Part model, mm, in its own coordinate system. Face numbers are marked on the shaded views. A direction names the side the tool comes from. Round coordinates to 2 decimals unless told otherwise and drop trailing zeros. Write each loop counter-clockwise with the first axis right and the second up, starting at its lowest first coordinate (ties: lowest second). Pieces come first, ordered by that corner, then holes. Notation, with made-up numbers: M 26.5,2.5 L 80.5,2.5 A15 cw 80.5,14.5 Z; hole C -9.5,-35.75 d7. An arc over 180 degrees is marked long. Answer as a JSON object with one key per item and string values. Group by question number.
1. Band-saw the part on D-D, the plane x = -11. Write the cut outline in (y, z), plus the area to 3 significant figures.
2. Band-saw the part on A-A, the plane y = -56.5. Write the cut outline in (x, z).
3. Drop flat-ended pins along their axis: pin 1 (5 mm diameter, centred on x = -11, z = 34, fed in from -Y); pin 2 (4 mm diameter, centred on x = -23.5, y = -55.5, fed in from +Z); pin 3 (6 mm diameter, centred on x = -8.5, y = -39.5, fed in from +Z); pin 4 (2.5 mm diameter, centred on y = -56.5, z = 30, fed in from -X). Give the stop position or say it passes through.
4. Which spindle directions (+Z, -Z, +X, -X, +Y, -Y) get a long thin tool onto all of the face, cutting with end or side? Do the marked faces 1, 2, 3 and 4. Say none if no direction does.
5. Band-saw the part on C-C, the plane x = 26. Write the cut outline in (y, z).
6. Two-plate mould, pull along Y, no slides. Class the marked faces 5, 6, 7 and 8: +Y half, -Y half, draft (parallel to the pull), parting line (faces both ways), or undercut.
7. Drill centre lines: line 1 (Z direction, x = 42.35, y = -13); line 2 (Z direction, x = -11, y = -37.5); line 3 (X direction, y = -1.6, z = 65). Where is each one in solid material? Low to high. Write a range as from..to.
8. Band-saw the part on B-B, the plane z = 17. Write the cut outline in (x, y).
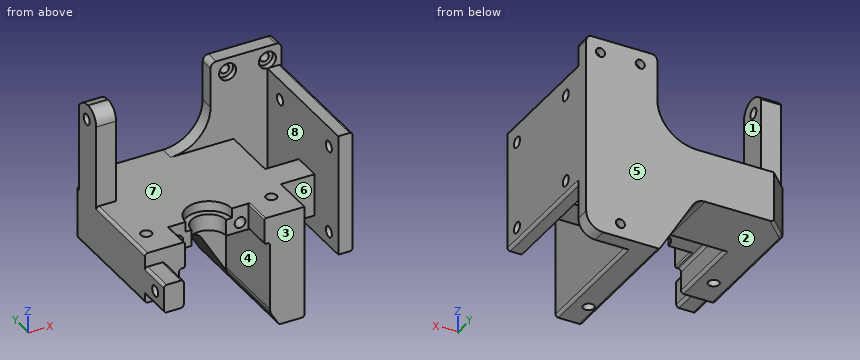
from build123d import *

# Parameters (mm, degrees)
PAD_DEPTH       = 70
SKETCH001_W     = 11.887794
SKETCH001_H     = 46.78
POCKET_DEPTH    = 70.001
POCKET001_DEPTH = 30
SKETCH003_R     = 1.9
POCKET002_DEPTH = 40.001
POCKET003_DEPTH = 3.5
POCKET004_DEPTH = 9
SKETCH021_W     = 28
SKETCH021_H     = 53.161749
POCKET005_DEPTH = 10
SKETCH022_W     = 32
SKETCH022_H     = 58.660217
POCKET006_DEPTH = 28
POCKET007_DEPTH = 51
SKETCH008_W     = 19.05323
SKETCH008_H     = 10.69447
SKETCH008_W_2   = 35.750058
SKETCH008_H_2   = 36.172176
POCKET008_DEPTH = 45
SKETCH009_R     = 1.9
POCKET009_DEPTH = 5
SKETCH015_W     = 11
SKETCH015_H     = 38.184422
SKETCH015_W_2   = 19.881198
SKETCH015_H_2   = 10
PAD001_DEPTH    = 7
SKETCH011_R     = 1.9
POCKET010_DEPTH = 10
SKETCH014_W     = 10
SKETCH014_H     = 15
PAD002_DEPTH    = 18
SKETCH010_R     = 1.6
POCKET011_DEPTH = 6
SKETCH017_R     = 3
POCKET012_DEPTH = 2
SKETCH013_R     = 1.9
POCKET013_DEPTH = 10
CHAMFER_SIZE    = 7
CHAMFER001_SIZE = 3
FILLET_R        = 6
FILLET001_R     = 5
FILLET002_R     = 1
FILLET003_R     = 1
FILLET004_R     = 1
FILLET005_R     = 1
FILLET006_R     = 5
FILLET007_R     = 4
FILLET008_R     = 1
FILLET009_R     = 1
FILLET010_R     = 1
FILLET011_R     = 0.5
FILLET012_R     = 1
FILLET013_R     = 1
FILLET014_R     = 1
FILLET015_R     = 14
FILLET016_R     = 2
FILLET017_R     = 6
FILLET018_R     = 1


with BuildPart() as part:
    # Sketch → Pad (new body)
    with BuildSketch(Plane.XY):
        Polygon((0, 0), (45, 0), (45, -50), (-28, -50), (-28, 0), align=None)
    extrude(amount=PAD_DEPTH)

    # Sketch001 (on Face7 of Pad) → Pocket (cut, through all)
    with BuildSketch(Plane.XY.offset(70)):
        with Locations((34.056103, -28.39)):
            Rectangle(SKETCH001_W, SKETCH001_H)
    extrude(amount=-POCKET_DEPTH, mode=Mode.SUBTRACT)

    # Sketch002 (on Face5 of Pocket) → Pocket001 (cut)
    with BuildSketch(Plane.XY.offset(70)):
        Polygon((30, -5), (30, -65.096024), (-40.783405, -65.096024), (-40.783405, 12.994774), (20, 12.994774), (20, -5), align=None)
    extrude(amount=-POCKET001_DEPTH, mode=Mode.SUBTRACT)

    # Sketch003 (on Face6 of Pocket001) → Pocket002 (cut, through all)
    with BuildSketch(Plane.XY.offset(40)):
        with Locations((-22, -40)):
            Circle(SKETCH003_R)
        with Locations((22, -40)):
            Circle(SKETCH003_R)
    extrude(amount=-POCKET002_DEPTH, mode=Mode.SUBTRACT)

    # Sketch004 (on Face6 of Pocket002) → Pocket003 (cut)
    with BuildSketch(Plane.XY.offset(40)):
        with BuildLine():
            ThreePointArc((8.125, -40), (0, -31.875), (-8.125, -40))
            Line((-8.125, -59.24), (-8.125, -40))
            Line((8.125, -59.24), (-8.125, -59.24))
            Line((8.125, -40), (8.125, -59.24))
        make_face()
    extrude(amount=-POCKET003_DEPTH, mode=Mode.SUBTRACT)

    # Sketch018 → Pocket004 (cut)
    with BuildSketch(Plane.XY.offset(36.5)):
        with BuildLine():
            ThreePointArc((6.1, -40), (0, -33.9), (-6.1, -40))
            Line((-6.1, -40), (-6.1, -58.98))
            Line((6.1, -58.98), (-6.1, -58.98))
            Line((6.1, -40), (6.1, -58.98))
        make_face()
    extrude(amount=-POCKET004_DEPTH, mode=Mode.SUBTRACT)

    # Sketch021 (on Face9 of Pocket004) → Pocket005 (cut)
    with BuildSketch(Plane.XZ.offset(50)):
        with Locations((0, 16.83664)):
            Rectangle(SKETCH021_W, SKETCH021_H)
    extrude(amount=-POCKET005_DEPTH, mode=Mode.SUBTRACT)

    # Sketch022 (on Face13 of Pocket005) → Pocket006 (cut)
    with BuildSketch(Plane.XZ.offset(50)):
        with Locations((0, 1.369891)):
            Rectangle(SKETCH022_W, SKETCH022_H)
    extrude(amount=-POCKET006_DEPTH, mode=Mode.SUBTRACT)

    # Sketch023 (on Face9 of Pocket006) → Pocket007 (cut)
    with BuildSketch(Plane.XZ.offset(50)):
        Polygon((-38.33, 22), (6, 22), (24, -8), (-38.33, -8), align=None)
    extrude(amount=-POCKET007_DEPTH, mode=Mode.SUBTRACT)

    # Sketch008 (on Face14 of Pocket007) → Pocket008 (cut)
    with BuildSketch(Plane.XZ.offset(50)):
        with Locations((44.142395, 67.347235)):
            Rectangle(SKETCH008_W, SKETCH008_H)
        with Locations((52.797694, 0.913912)):
            Rectangle(SKETCH008_W_2, SKETCH008_H_2)
    extrude(amount=-POCKET008_DEPTH, mode=Mode.SUBTRACT)

    # Sketch009 (on Face3 of Pocket008) → Pocket009 (cut)
    with BuildSketch(Plane.YZ.offset(45)):
        with Locations((-44, 55)):
            Circle(SKETCH009_R)
        with Locations((-13, 24)):
            Circle(SKETCH009_R)
        with Locations((-13, 55)):
            Circle(SKETCH009_R)
        with Locations((-44, 24)):
            Circle(SKETCH009_R)
    extrude(amount=-POCKET009_DEPTH, mode=Mode.SUBTRACT)

    # Sketch015 (on Face27 of Pocket009) → Pad001 (join)
    with BuildSketch(Plane(origin=(-28, 0, 0), x_dir=(0, -1, 0), z_dir=(-1, 0, 0))):
        with Locations((13.5, 54.907789)):
            Rectangle(SKETCH015_W, SKETCH015_H)
        with Locations((52.059401, 30)):
            Rectangle(SKETCH015_W_2, SKETCH015_H_2)
    extrude(amount=-PAD001_DEPTH)

    # Sketch011 (on Face27 of Pad001) → Pocket010 (cut)
    with BuildSketch(Plane(origin=(-28, 0, 0), x_dir=(0, -1, 0), z_dir=(-1, 0, 0))):
        with Locations((56.5, 30)):
            Circle(SKETCH011_R)
        with Locations((13, 68.5)):
            Circle(SKETCH011_R)
    extrude(amount=-POCKET010_DEPTH, mode=Mode.SUBTRACT)

    # Sketch014 (on Face3 of Pocket010) → Pad002 (join)
    with BuildSketch(Plane.YZ.offset(45)):
        with Locations((-30, 32.5)):
            Rectangle(SKETCH014_W, SKETCH014_H)
    extrude(amount=-PAD002_DEPTH)

    # Sketch010 → Pocket011 (cut)
    with BuildSketch(Plane(origin=(0, 0, 0), x_dir=(-1, 0, 0), z_dir=(0, 1, 0))):
        with Locations((-33, 5)):
            Circle(SKETCH010_R)
        with Locations((-40, 65)):
            Circle(SKETCH010_R)
        with Locations((-26, 65)):
            Circle(SKETCH010_R)
    extrude(amount=-POCKET011_DEPTH, mode=Mode.SUBTRACT)

    # Sketch017 (on Face34 of Pocket011) → Pocket012 (cut)
    with BuildSketch(Plane.XZ.offset(5)):
        with Locations((26, 65)):
            Circle(SKETCH017_R)
        with Locations((33, 5)):
            Circle(SKETCH017_R)
        with Locations((40, 65)):
            Circle(SKETCH017_R)
    extrude(amount=-POCKET012_DEPTH, mode=Mode.SUBTRACT)

    # Sketch013 (on Face43 of Pocket012) → Pocket013 (cut)
    with BuildSketch(Plane.XZ.offset(40)):
        with Locations((-11, 34)):
            Circle(SKETCH013_R)
        with Locations((11, 34)):
            Circle(SKETCH013_R)
    extrude(amount=-POCKET013_DEPTH, mode=Mode.SUBTRACT)

    # Chamfer
    chamfer_edges = [part.edges().sort_by_distance(p)[0] for p in [
        (-28, 0, 31),
    ]]
    chamfer(chamfer_edges, length=CHAMFER_SIZE)

    # Chamfer001
    chamfer001_edges = [part.edges().sort_by_distance(p)[0] for p in [
        (-24.5, -8, 74),
    ]]
    chamfer(chamfer001_edges, length=CHAMFER001_SIZE)

    # Fillet
    fillet_edges = [part.edges().sort_by_distance(p)[0] for p in [
        (-24.5, -11, 74),
    ]]
    fillet(fillet_edges, radius=FILLET_R)

    # Fillet001
    fillet001_edges = [part.edges().sort_by_distance(p)[0] for p in [
        (-24.5, -19, 74),
    ]]
    fillet(fillet001_edges, radius=FILLET001_R)

    # Fillet002
    fillet002_edges = [part.edges().sort_by_distance(p)[0] for p in [
        (-28, -34.5, 40),
    ]]
    fillet(fillet002_edges, radius=FILLET002_R)

    # Fillet003
    fillet003_edges = [part.edges().sort_by_distance(p)[0] for p in [
        (-28, -28.5, 22),
    ]]
    fillet(fillet003_edges, radius=FILLET003_R)

    # Fillet004
    fillet004_edges = [part.edges().sort_by_distance(p)[0] for p in [
        (-16, -36, 22),
    ]]
    fillet(fillet004_edges, radius=FILLET004_R)

    # Fillet005
    fillet005_edges = [part.edges().sort_by_distance(p)[0] for p in [
        (19.2, -25, 0),
    ]]
    fillet(fillet005_edges, radius=FILLET005_R)

    # Fillet006
    fillet006_edges = [part.edges().sort_by_distance(p)[0] for p in [
        (6, -11, 22),
    ]]
    fillet(fillet006_edges, radius=FILLET006_R)

    # Fillet007
    fillet007_edges = [part.edges().sort_by_distance(p)[0] for p in [
        (16, -36, 5.333333),
    ]]
    fillet(fillet007_edges, radius=FILLET007_R)

    # Fillet008
    fillet008_edges = [part.edges().sort_by_distance(p)[0] for p in [
        (16, -36, 30.7),
    ]]
    fillet(fillet008_edges, radius=FILLET008_R)

    # Fillet009
    fillet009_edges = [part.edges().sort_by_distance(p)[0] for p in [
        (-16, -36, 30.7),
    ]]
    fillet(fillet009_edges, radius=FILLET009_R)

    # Fillet010
    fillet010_edges = [part.edges().sort_by_distance(p)[0] for p in [
        (-28, -56, 25),
        (-21, -56, 25),
        (-21, -56, 35),
        (-28, -56, 35),
    ]]
    fillet(fillet010_edges, radius=FILLET010_R)

    # Fillet011
    fillet011_edges = [part.edges().sort_by_distance(p)[0] for p in [
        (14, -45, 30.7),
        (-14, -45, 30.7),
        (14, -45, 40),
        (-14, -45, 40),
    ]]
    fillet(fillet011_edges, radius=FILLET011_R)

    # Fillet012
    fillet012_edges = [part.edges().sort_by_distance(p)[0] for p in [
        (28.112206, -27.5, 0),
    ]]
    fillet(fillet012_edges, radius=FILLET012_R)

    # Fillet013
    fillet013_edges = [part.edges().sort_by_distance(p)[0] for p in [
        (45, -27.5, 19),
    ]]
    fillet(fillet013_edges, radius=FILLET013_R)

    # Fillet014
    fillet014_edges = [part.edges().sort_by_distance(p)[0] for p in [
        (45, -27.5, 62),
    ]]
    fillet(fillet014_edges, radius=FILLET014_R)

    # Fillet015
    fillet015_edges = [part.edges().sort_by_distance(p)[0] for p in [
        (20, -2.5, 40),
    ]]
    fillet(fillet015_edges, radius=FILLET015_R)

    # Fillet016
    fillet016_edges = [part.edges().sort_by_distance(p)[0] for p in [
        (20, -2.5, 70),
        (45, -2.5, 70),
    ]]
    fillet(fillet016_edges, radius=FILLET016_R)

    # Fillet017
    fillet017_edges = [part.edges().sort_by_distance(p)[0] for p in [
        (45, -2.5, 0),
    ]]
    fillet(fillet017_edges, radius=FILLET017_R)

    # Fillet018
    fillet018_edges = [part.edges().sort_by_distance(p)[0] for p in [
        (-28, -7, 31.5),
    ]]
    fillet(fillet018_edges, radius=FILLET018_R)


solid = part.part
Worked answers:
{
 "1": {"outline": "M -40,30.7 L -22,30.7 L -22,22 L 0,22 L 0,40 L -40,40 L -40,35.9 L -30,35.9 L -30,32.1 L -40,32.1 Z", "area": "525 mm^2"},
 "2": {"outline": "M -28,26 A1 ccw -27,25 L -22,25 A1 ccw -21,26 L -21,28.1 L -28,28.1 Z; M -28,31.9 L -21,31.9 L -21,34 A1 ccw -22,35 L -27,35 A1 ccw -28,34 Z"},
 "3": {"pin 1": "stops at y = -40", "pin 2": "stops at z = 35", "pin 3": "stops at z = 40", "pin 4": "passes through"},
 "4": {"face 1": "+Z, +Y, -Y", "face 2": "-Z, -X, +Y, -Y", "face 3": "+Z, -Z, +X, -Y", "face 4": "-Z, -Y"},
 "5": {"outline": "M -50,0 L 0,0 L 0,63.4 L -3,63.4 L -3,62 L -5,62 L -5,40 L -50,40 Z; M -5,68 L -3,68 L -3,66.6 L 0,66.6 L 0,70 L -5,70 Z"},
 "6": {"face 5": "+Y half", "face 6": "-Y half", "face 7": "draft", "face 8": "undercut"},
 "7": {"line 1": "z = 19..22.1, 25.9..53.1, 56.9..62", "line 2": "z = 30.7..32.1, 35.9..40", "line 3": "x = 20..24.4, 27.6..38.4, 41.6..45"},
 "8": {"outline": "M 9,-22 L 16,-22 L 16,-50 L 28.11,-50 L 28.11,-5 L 45,-5 L 45,0 L 9,0 Z; hole C 22,-40 d3.8"}
}
